from build123d import *

# Parameters (mm, degrees)
SKETCH3_R               = 10
CUT_EXTRUDE1_DEPTH      = 307.30866785
CIRPATTERN1_COUNT       = 6
SKETCH5_R               = 100
BOSS_EXTRUDE1_DEPTH     = 10
CUT_EXTRUDE2_DEPTH      = 325.191301549
CUT_EXTRUDE2_DEPTH_BACK = 325.191301549
SKETCH4_W               = 32
SKETCH4_H               = 10
CUT_EXTRUDE4_DEPTH      = 329.329103188
CUT_EXTRUDE4_DEPTH_BACK = 329.329103188
SKETCH6_R               = 52.5


with BuildPart() as part:
    # Sketch2 → Revolve1 (revolve)
    with BuildSketch(Plane(origin=(0, 0, 0), x_dir=(-1, 0, 0), z_dir=(0, 1, 0))):
        Polygon((-138.434782609, 52.5), (-268.434782609, 52.5), (-268.434782609, 105), (-193.434782609, 105), (-193.434782609, 185), (-218.434782609, 185), (-218.434782609, 210), (-138.434782609, 210), align=None)
    revolve(axis=Axis((0, 0, 0), (1, 0, 0)))

    # Sketch3 → Cut-Extrude1 (cut, through all)
    with BuildSketch(Plane.YZ.offset(193.434782609)):
        with Locations(Location((0, 145, 0), (0, 0, 270))):
            Circle(SKETCH3_R)
    cut_extrude1 = extrude(amount=-CUT_EXTRUDE1_DEPTH, mode=Mode.SUBTRACT)

    # CirPattern1: Cut-Extrude1 ×6 about axis
    cirpattern1_axis = Axis((0, 0, 0), (1, 0, 0))
    for i in range(1, CIRPATTERN1_COUNT):
        add(cut_extrude1.rotate(cirpattern1_axis, i * 360 / CIRPATTERN1_COUNT), mode=Mode.SUBTRACT)

    # Sketch5 → Boss-Extrude1 (add)
    with BuildSketch(Plane(origin=(138.434782609, 0, 0), x_dir=(0, -1, 0), z_dir=(-1, 0, 0))):
        with Locations(Location((0, 0, 0), (0, 0, 90))):
            Circle(SKETCH5_R)
    extrude(amount=BOSS_EXTRUDE1_DEPTH)

    # Sketch4 → Cut-Extrude2 (cut, two sides: drawn at the far end of the back side and taken through both)
    with BuildSketch(Plane(origin=(138.434782609, 0, 0), x_dir=(0, -1, 0), z_dir=(-1, 0, 0)).offset(-CUT_EXTRUDE2_DEPTH_BACK)):
        with Locations((0, 55.002499938)):
            Rectangle(SKETCH4_W, SKETCH4_H)
    extrude(amount=CUT_EXTRUDE2_DEPTH + CUT_EXTRUDE2_DEPTH_BACK, mode=Mode.SUBTRACT)

    # Sketch6 → Cut-Extrude4 (cut, two sides: drawn at the far end of the back side and taken through both)
    with BuildSketch(Plane(origin=(128.434782609, 0, 0), x_dir=(0, -1, 0), z_dir=(-1, 0, 0)).offset(-CUT_EXTRUDE4_DEPTH_BACK)):
        Circle(SKETCH6_R)
    extrude(amount=CUT_EXTRUDE4_DEPTH + CUT_EXTRUDE4_DEPTH_BACK, mode=Mode.SUBTRACT)


solid = part.part
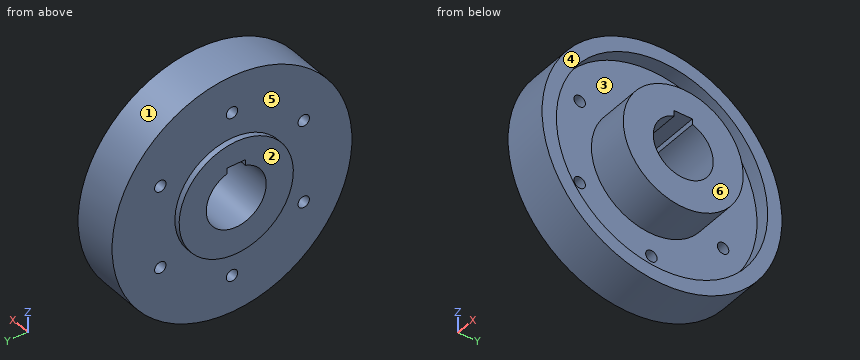
Source: CAD feature listing. Evaluate the final solid. Frame: model axes, mm. Face numbers are marked on the shaded views. A direction names the side the tool comes from. Round coordinates to 2 decimals unless told otherwise and drop trailing zeros. Loops run counter-clockwise (first coordinate to the right, second up) from the corner with the lowest first, then second, coordinate; pieces in that order, holes last. Notation, with made-up numbers: (82, -14) - (141, -14) arc R16 ccw to (141, -5) - close; hole circle Ø5 at (29.5, 53.25). An arc over 180 degrees is marked (long way). Write item = value, one per line. Start each with the question number.
(1) Section query A-A, the plane x = 201.5. Output: boundary loops of the cut face in (y, z), plus the area to 3 significant figures.
(2) Set-up query: the marked faces 4, 5 and 6. Return all of +Z, -Z, +X, -X, +Y, -Y with unobstructed straight access to the full face (end or side cutting, diameter ignored); none if empty.
(3) Ray query, line 1 along Z through (x, y) = (221, 0); line 2 along Z through (x, y) = (216.5, 3.5); line 3 along Y through (x, z) = (156, -72). Return the intervals inside material, ascending. Write a range as from..to.
(4) Pin query (flat end, axial travel): pin 1 (10 mm diameter, centred on x = 151, y = 124.5, fed in from +Z); pin 2 (23 mm diameter, centred on y = 0, z = -145, fed in from +X); pin 3 (12 mm diameter, centred on y = -125.57, z = 72.5, fed in from +X); pin 4 (9.5 mm diameter, centred on x = 175, y = -5, fed in from -Z). Return the tip coordinate at first contact, or that it passes through.
(5) Section query D-D, the plane z = 72.5. Output: boundary loops of the cut face in (x, y).
(6) Section query C-C, the plane z = -18. Output: boundary loops of the cut face in (x, y).
(7) Pull-direction query (Z, two-part tool) for the marked faces 1, 2 and 3; classes: +Z half, -Z half, draft (parallel to the pull), parting line (faces both ways), or undercut.
(8) Section query B-B, the plane y = 0. Output: boundary loops of the cut face in (x, z).
Conclusion:
q1.outline = circle Ø420 at (0, 0); circle Ø210 at (0, 0); hole circle Ø370 at (0, 0); hole (-16, 50) arc R52.5 ccw (long way) to (16, 50) - (16, 60) - (-16, 60) - close
q1.area = 56,700 mm2
q2.face_4 = +X
q2.face_5 = -X
q2.face_6 = +Z, -Z, +X, +Y, -Y
q3.line_1 = -105..-52.5, 60..105
q3.line_2 = -209.97..-184.97, -104.94..-52.38, 60..104.94, 184.97..209.97
q3.line_3 = -197.27..-135.56, -115.59..115.59, 135.56..197.27
q4.pin_1 = 172.68
q4.pin_2 = 193.43
q4.pin_3 = through
q4.pin_4 = -210
q5.outline = (128.43, -68.87) - (138.43, -68.87) - (138.43, -115.57) - (193.43, -115.57) - (193.43, -75.95) - (268.43, -75.95) - (268.43, 75.95) - (193.43, 75.95) - (193.43, 115.57) - (138.43, 115.57) - (138.43, 68.87) - (128.43, 68.87) - close; (138.43, -197.09) - (218.43, -197.09) - (218.43, -170.2) - (193.43, -170.2) - (193.43, -135.57) - (138.43, -135.57) - close; (138.43, 135.57) - (193.43, 135.57) - (193.43, 170.2) - (218.43, 170.2) - (218.43, 197.09) - (138.43, 197.09) - close
q6.outline = (128.43, -98.37) - (138.43, -98.37) - (138.43, -209.23) - (218.43, -209.23) - (218.43, -184.12) - (193.43, -184.12) - (193.43, -103.45) - (268.43, -103.45) - (268.43, -49.32) - (128.43, -49.32) - close; (128.43, 49.32) - (268.43, 49.32) - (268.43, 103.45) - (193.43, 103.45) - (193.43, 184.12) - (218.43, 184.12) - (218.43, 209.23) - (138.43, 209.23) - (138.43, 98.37) - (128.43, 98.37) - close
q7.face_1 = parting line
q7.face_2 = draft
q7.face_3 = undercut
q8.outline = (128.43, -100) - (138.43, -100) - (138.43, -135) - (193.43, -135) - (193.43, -105) - (268.43, -105) - (268.43, -52.5) - (128.43, -52.5) - close; (128.43, 60) - (268.43, 60) - (268.43, 105) - (193.43, 105) - (193.43, 135) - (138.43, 135) - (138.43, 100) - (128.43, 100) - close; (138.43, -210) - (218.43, -210) - (218.43, -185) - (193.43, -185) - (193.43, -155) - (138.43, -155) - close; (138.43, 155) - (193.43, 155) - (193.43, 185) - (218.43, 185) - (218.43, 210) - (138.43, 210) - close
